Here's how the part is built. I have some questions about the finished solid (model axes, mm). Round coordinates to 2 decimals unless told otherwise and drop trailing zeros. Loops run counter-clockwise (first coordinate to the right, second up) from the corner with the lowest first, then second, coordinate; pieces in that order, holes last. Notation, with made-up numbers: M 80.25,26 L 107.25,26 A18 cw 107.25,46 Z; hole C 56.25,70.25 d11. An arc over 180 degrees is marked long. Answer as a JSON object with one key per item and string values.
from build123d import *

# Parameters (mm, degrees)
SKETCH1_W           = 6.27
SKETCH1_H           = 1.37
SKETCH1_R           = 1.25
SKETCH1_W_2         = 5.63
SKETCH1_H_2         = 0.85
SKETCH1_R_2         = 0.685
SKETCH1_R_3         = 0.5
SKETCH1_W_3         = 1.34
SKETCH1_H_3         = 0.3
SKETCH1_W_4         = 2.76
BOSS_EXTRUDE2_DEPTH = 0.5
SKETCH4_R           = 0.5
BOSS_EXTRUDE3_DEPTH = 1.41
SKETCH5_R           = 0.5
BOSS_EXTRUDE4_DEPTH = 1.41
SKETCH6_W           = 6.27
SKETCH6_H           = 1.37
BOSS_EXTRUDE5_DEPTH = 0.8
SKETCH7_W           = 1.34
SKETCH7_H           = 0.3
SKETCH7_W_2         = 2.76
BOSS_EXTRUDE6_DEPTH = 5.5
SKETCH8_W           = 1.38
SKETCH8_H           = 2.92
CUT_EXTRUDE1_DEPTH  = 5.5
SKETCH9_R           = 0.4
CUT_EXTRUDE2_DEPTH  = 5.5
SKETCH10_R          = 0.4
CUT_EXTRUDE4_DEPTH  = 5.5
SKETCH11_W          = 0.8
SKETCH11_H          = 0.5
BOSS_EXTRUDE7_DEPTH = 5
SKETCH12_W          = 0.8
SKETCH12_H          = 0.5
BOSS_EXTRUDE8_DEPTH = 5


with BuildPart() as part:
    # Sketch1 → Boss-Extrude2 (new body)
    # profile 1 of 9: a face of its own
    with BuildSketch(Plane(origin=(0, 0, 0), x_dir=(1, 0, 0), z_dir=(0, 1, 0))):
        with BuildLine():
            Line((0, 5.31), (0, 5.14))
            ThreePointArc((0, 5.14), (-0.527207794, 3.867207794), (-1.8, 3.34))
            Line((-1.8, 3.34), (-12.035, 3.34))
            ThreePointArc((-12.035, 3.34), (-11.550631855, 3.139368145), (-11.35, 2.655))
            ThreePointArc((-11.35, 2.655), (-11.550631855, 2.170631855), (-12.035, 1.97))
            Line((-12.035, 1.97), (-1.8, 1.97))
            ThreePointArc((-1.8, 1.97), (-0.527207794, 1.442792206), (0, 0.17))
            Line((0, 0.17), (0, 0))
            Line((0, 0), (0.77, 0))
            Line((0.77, 0), (1.61, 0))
            Line((1.61, 0), (17.61, 0))
            Line((17.61, 0), (17.61, 8.51))
            Line((17.61, 8.51), (14.85, 8.51))
            Line((14.85, 8.51), (9.04, 8.51))
            Line((9.04, 8.51), (7.7, 8.51))
            Line((7.7, 8.51), (7.7, 5.31))
            Line((7.7, 5.31), (1.61, 5.31))
            Line((1.61, 5.31), (0.77, 5.31))
            Line((0.77, 5.31), (0, 5.31))
        make_face()
        with Locations((10.655, 1.325)):
            Rectangle(SKETCH1_W, SKETCH1_H, mode=Mode.SUBTRACT)
        with Locations(Location((1.31, 2.655, 0), (0, 0, 270))):
            Circle(SKETCH1_R, mode=Mode.SUBTRACT)
        with Locations((10.655, 3.795)):
            Rectangle(SKETCH1_W, SKETCH1_H, mode=Mode.SUBTRACT)
        with Locations(Location((16.06, 2.655, 0), (0, 0, 270))):
            Circle(SKETCH1_R, mode=Mode.SUBTRACT)
        with Locations((10.615, 5.875)):
            Rectangle(SKETCH1_W_2, SKETCH1_H_2, mode=Mode.SUBTRACT)
    # profile 2 of 9: a face of its own
    with BuildSketch(Plane(origin=(0, 0, 0), x_dir=(1, 0, 0), z_dir=(0, 1, 0))):
        with BuildLine():
            Line((0.77, 11.64), (0.77, 5.31))
            Line((0.77, 5.31), (1.61, 5.31))
            Line((1.61, 5.31), (1.61, 11.64))
            ThreePointArc((1.61, 11.64), (1.363969696, 12.233969696), (0.77, 12.48))
            Line((0.77, 12.48), (-17.73, 12.48))
            Line((-17.73, 12.48), (-17.73, 11.64))
            Line((-17.73, 11.64), (0.77, 11.64))
        make_face()
    # profile 3 of 9: a face of its own
    with BuildSketch(Plane(origin=(0, 0, 0), x_dir=(1, 0, 0), z_dir=(0, 1, 0))):
        with BuildLine():
            Line((1.61, 0), (0.77, 0))
            Line((0.77, 0), (0.77, -6.33))
            Line((0.77, -6.33), (-17.73, -6.33))
            Line((-17.73, -6.33), (-17.73, -7.17))
            Line((-17.73, -7.17), (0.77, -7.17))
            ThreePointArc((0.77, -7.17), (1.363969696, -6.923969696), (1.61, -6.33))
            Line((1.61, -6.33), (1.61, 0))
        make_face()
    # profile 4 of 9: a face of its own
    with BuildSketch(Plane(origin=(0, 0, 0), x_dir=(1, 0, 0), z_dir=(0, 1, 0))):
        with Locations((10.655, 1.325)):
            Rectangle(SKETCH1_W, SKETCH1_H)
    # profile 5 of 9: a face of its own
    with BuildSketch(Plane(origin=(0, 0, 0), x_dir=(1, 0, 0), z_dir=(0, 1, 0))):
        with Locations((10.655, 3.795)):
            Rectangle(SKETCH1_W, SKETCH1_H)
    # profile 6 of 9: a face of its own
    with BuildSketch(Plane(origin=(0, 0, 0), x_dir=(1, 0, 0), z_dir=(0, 1, 0))):
        with Locations((-12.035, 2.655)):
            Circle(SKETCH1_R_2)
        with Locations((-12.035, 2.655)):
            Circle(SKETCH1_R_3, mode=Mode.SUBTRACT)
    # profile 7 of 9: a face of its own
    with BuildSketch(Plane(origin=(0, 0, 0), x_dir=(1, 0, 0), z_dir=(0, 1, 0))):
        with Locations((-12.035, 2.655)):
            Circle(SKETCH1_R_3)
    # profile 8 of 9: a face of its own
    with BuildSketch(Plane(origin=(0, 0, 0), x_dir=(1, 0, 0), z_dir=(0, 1, 0))):
        with Locations((8.37, 8.66)):
            Rectangle(SKETCH1_W_3, SKETCH1_H_3)
    # profile 9 of 9: a face of its own
    with BuildSketch(Plane(origin=(0, 0, 0), x_dir=(1, 0, 0), z_dir=(0, 1, 0))):
        with Locations((16.23, 8.66)):
            Rectangle(SKETCH1_W_4, SKETCH1_H_3)
    extrude(amount=BOSS_EXTRUDE2_DEPTH)

    # Sketch4 → Boss-Extrude3 (add)
    with BuildSketch(Plane(origin=(0, 0.5, 0), x_dir=(1, 0, 0), z_dir=(0, 1, 0))):
        with Locations(Location((-12.040018383, 2.65, 0), (0, 0, 270))):
            Circle(SKETCH4_R)
    extrude(amount=BOSS_EXTRUDE3_DEPTH)

    # Sketch5 → Boss-Extrude4 (add)
    with BuildSketch(Plane.XZ):
        with Locations(Location((-12.04, -2.66, 0), (0, 0, 90))):
            Circle(SKETCH5_R)
    extrude(amount=BOSS_EXTRUDE4_DEPTH)

    # Sketch6 → Boss-Extrude5 (add)
    with BuildSketch(Plane(origin=(0, 0.5, 0), x_dir=(1, 0, 0), z_dir=(0, 1, 0))):
        with Locations((10.655, 3.795)):
            Rectangle(SKETCH6_W, SKETCH6_H)
        with Locations((10.655, 1.325)):
            Rectangle(SKETCH6_W, SKETCH6_H)
    extrude(amount=BOSS_EXTRUDE5_DEPTH)

    # Sketch7 → Boss-Extrude6 (add)
    with BuildSketch(Plane(origin=(0, 0.5, 0), x_dir=(1, 0, 0), z_dir=(0, 1, 0))):
        with Locations((8.37, 8.66)):
            Rectangle(SKETCH7_W, SKETCH7_H)
        with Locations((16.23, 8.66)):
            Rectangle(SKETCH7_W_2, SKETCH7_H)
    extrude(amount=BOSS_EXTRUDE6_DEPTH)

    # Sketch8 → Cut-Extrude1 (cut)
    with BuildSketch(Plane.XY.offset(-8.51)):
        with Locations((15.54, 3.06)):
            Rectangle(SKETCH8_W, SKETCH8_H)
    extrude(amount=-CUT_EXTRUDE1_DEPTH, mode=Mode.SUBTRACT)

    # Sketch9 → Cut-Extrude2 (cut)
    with BuildSketch(Plane.XY.offset(-8.51)):
        with BuildLine():
            ThreePointArc((7.7, 5.2), (7.934314575, 5.765685425), (8.5, 6))
            Line((8.5, 6), (7.7, 6))
            Line((7.7, 6), (7.7, 5.2))
        make_face()
        with Locations((8.58, 4.82)):
            Circle(SKETCH9_R)
        with Locations((8.58, 1.32)):
            Circle(SKETCH9_R)
    extrude(amount=-CUT_EXTRUDE2_DEPTH, mode=Mode.SUBTRACT)

    # Sketch10 → Cut-Extrude4 (cut)
    with BuildSketch(Plane.XY.offset(-8.51)):
        with Locations((16.59, 4.82)):
            Circle(SKETCH10_R)
        with BuildLine():
            Line((17.61, 6), (16.81, 6))
            ThreePointArc((16.81, 6), (17.375685425, 5.765685425), (17.61, 5.2))
            Line((17.61, 5.2), (17.61, 6))
        make_face()
        with Locations((16.59, 1.32)):
            Circle(SKETCH10_R)
    extrude(amount=-CUT_EXTRUDE4_DEPTH, mode=Mode.SUBTRACT)

    # Sketch11 → Boss-Extrude7 (add)
    with BuildSketch(Plane.XY.offset(-1.97)):
        with Locations((-3.2, 0.25)):
            Rectangle(SKETCH11_W, SKETCH11_H)
    extrude(amount=BOSS_EXTRUDE7_DEPTH)

    # Sketch12 → Boss-Extrude8 (add)
    with BuildSketch(Plane(origin=(0, 0, -3.34), x_dir=(-1, 0, 0), z_dir=(0, 0, -1))):
        with Locations((3.2, 0.25)):
            Rectangle(SKETCH12_W, SKETCH12_H)
    extrude(amount=BOSS_EXTRUDE8_DEPTH)


solid = part.part
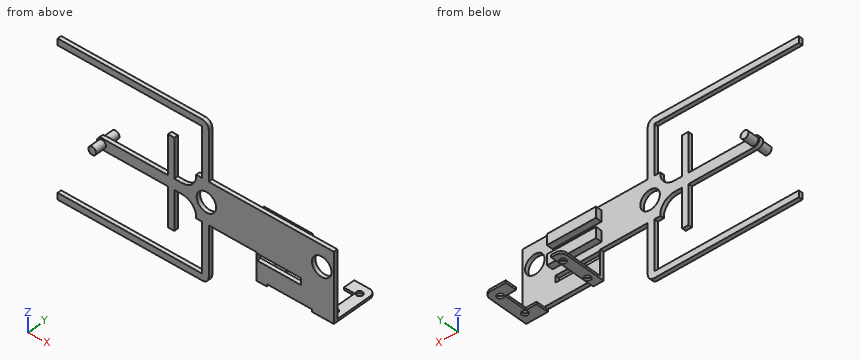
Item 1: Please list where these lines run through material, in increasing order: probe 1 along Y at (x, z) = (16.59, -8.6); probe 2 along Y at (x, z) = (1, -6.5). Write a range as from..to.
Resolved:
{"probe 1": "0..0.92, 1.72..4.42, 5.22..6", "probe 2": "0..0.5"}
Item 2: I want a section at D-D, the plane z = -2.66. Please give me the cut outline in (x, y).
Resolved:
{"outline": "M -12.72,0 L -12.54,0 L -12.54,-1.41 L -11.54,-1.41 L -11.54,0 L 0.06,0 L 0.06,0.5 L -11.54,0.5 L -11.54,1.91 L -12.54,1.91 L -12.54,0.5 L -12.72,0.5 Z; M 2.56,0 L 14.81,0 L 14.81,0.5 L 2.56,0.5 Z; M 17.31,0 L 17.61,0 L 17.61,0.5 L 17.31,0.5 Z"}
Item 3: I want a section at C-C, the plane y = 2.75. Please give me the cut outline in (x, z), then the cut area to 3 significant figures.
Resolved:
{"outline": "M 7.7,-8.81 L 9.04,-8.81 L 9.04,-8.51 L 7.7,-8.51 Z; M 16.23,-8.81 L 17.61,-8.81 L 17.61,-8.51 L 16.23,-8.51 Z", "area": "0.816 mm²"}
Item 4: I want a section at A-A, the plane x = -8.5. Please give me the cut outline in (y, z).
Resolved:
{"outline": "M 0,-12.48 L 0.5,-12.48 L 0.5,-11.64 L 0,-11.64 Z; M 0,-3.34 L 0.5,-3.34 L 0.5,-1.97 L 0,-1.97 Z; M 0,6.33 L 0.5,6.33 L 0.5,7.17 L 0,7.17 Z"}
Item 5: I want a section at B-B, the plane z = 1. Please give me the cut outline in (x, y).
Resolved:
{"outline": "M -3.6,0 L -2.8,0 L -2.8,0.5 L -3.6,0.5 Z; M 0.77,0 L 1.61,0 L 1.61,0.5 L 0.77,0.5 Z"}
Item 6: I'm going to push flat-ended pins straight in: pin 1 Ø0.9 at (y, z) = (0.5, -3.5) entering from -X; pin 2 Ø2 at (x, y) = (17, 3) entering from -Z; pin 3 Ø3 at (x, y) = (16, 3.5) entering from +Z. Where does each tip first touch, or does it pass through?
Resolved:
{"pin 1": "x = -12.59", "pin 2": "z = -8.81", "pin 3": "z = -8.51"}
